Could you check a few things on this model? Use its own coordinates, in mm. A direction names the side the tool comes from. Give positions to 0.01 mm unless a question says otherwise; leave off trailing zeros. Loops run counter-clockwise (first coordinate to the right, second up) from the corner with the lowest first, then second, coordinate; pieces in that order, holes last. Notation, with made-up numbers: M -3.75,-3.5 L 33.25,-3.5 A24 ccw 33.25,16.5 Z; hole C 46,1 d5. An arc over 180 degrees is marked long. Answer in a Markdown table with one row per item. Add a question column.
1. Thinking about a two-plate mould opening in Z: for faces 3 (the flat face through (3, 148, -15)), 4 (the cylindrical face through (16.226, 117.044, -28.521)), 5 (the flat face through (15, 148, 0)), which applies, released by +Z, released by -Z, zero draft, split by the parting line, or undercut?
2. I'm going to push flat-ended pins straight in: pin 1 Ø10 at (y, z) = (254, -4) entering from -X; pin 2 Ø3 at (y, z) = (60, -15) entering from -X. Where does each tip first touch, or does it pass through?
3. If we section it at B-B on x = 23.75: List the corners of the cut face in (y, z) for me, then the cut area to 3 significant figures.
4. If we section it at A-A on y = 140: List the corners of the cut face in (x, z) for me, then the cut area to 3 significant figures.
5. I need wall thicknesses on line 1 along Y through (x, z) = (28.55, -15); line 2 along X through (y, z) = (227.5, -15.25); line 3 along Z through (x, y) = (15.5, 177). Which ranges of each line are inside material? Lowest first, please. Write a range as from..to.
6. Which directions (+Z, -Z, +X, -X, +Y, -Y) give clear straight access to the entire face, cutting with the end or side of a thin tool? Please do faces 1 (the flat face through (15, 148, -3)), 2 (the cylindrical face through (16.226, 117.044, -1.521)).
7. If we section it at D-D on y = 256: List the corners of the cut face in (x, z) for me, then the cut area to 3 significant figures.
8. If we section it at C-C on z = -22.75: List the corners of the cut face in (x, y) for me, then the cut area to 3 significant figures.
Autodesk Inventor part; units mm, degrees
ref_plane "YZ Plane" through (0, 0, 0) normal (1, 0, 0) x (0, 1, 0)
ref_plane "XZ Plane" through (0, 0, 0) normal (0, 1, 0) x (-1, 0, 0)
ref_plane "XY Plane" through (0, 0, 0) normal (0, 0, 1) x (1, 0, 0)
sketch "スケッチ1" plane through (0, 0, 0) normal (0, 1, 0) x (-1, 0, 0)
  line L0 (0, 0) -> (-30, 0)
  line L1 (-30, 0) -> (-30, -30)
  line L2 (-30, -30) -> (0, -30)
  line L3 (0, -30) -> (0, 0)
  line L4 (-3, -3) -> (-27, -3)
  line L5 (-27, -3) -> (-27, -27)
  line L6 (-27, -27) -> (-3, -27)
  line L7 (-3, -27) -> (-3, -3)
  dimension "d0" = 30
  dimension "d1" = 30
  dimension "d2" = 24
  dimension "d3" = 24
  dimension "d4" = 3
  dimension "d5" = 3
extrude "押し出し1" add sketch "スケッチ1" along normal blind 300
sketch "スケッチ2" plane through (0, 0, 0) normal (0, 0, 1) x (1, 0, 0)
  point P0 (0, 0)
  point P1 (13.8561, 31.5859)
sketch "スケッチ3" plane through (30, 0, 0) normal (1, 0, 0) x (0, 0, -1)
  line L0 (30, 0) -> (30, 300)
  line L1 (0, 0) -> (30, 0)
  point P0 (15, 60)
  point P1 (15, 30)
  point P2 (15, 0)
  dimension "d11" = 30
  dimension "d12" = 30
hole "穴1" at (30, 30, -15) at (30, 60, -15) direction (-1, 0, 0) diameter 3.2 end through all
sketch "スケッチ4" plane through (0, 0, 0) normal (0, 0, 1) x (1, 0, 0)
  line L0 (30, 0) -> (0, 0) construction
  line L1 (15, 0) -> (15, 300) construction
  line L2 (30, 300) -> (0, 300) construction
  point P0 (15, 120)
  point P1 (15, 140)
  dimension "d20" = 120
  dimension "d21" = 20
hole "穴2" at (15, 120, 0) at (15, 140, 0) direction (0, 0, -1) diameter 6.4 end through all
properties part number "base" material "アルミニウム 6061"
Results:
| question | item | result |
|---|---|---|
| 1 | face 3 | undercut |
| 1 | face 4 | zero draft |
| 1 | face 5 | released by +Z |
| 2 | pin 1 | x = 0 |
| 2 | pin 2 | through |
| 3 | outline | M 0,-30 L 300,-30 L 300,-27 L 0,-27 Z; M 0,-3 L 300,-3 L 300,0 L 0,0 Z |
| 3 | area | 1,800 mm2 |
| 4 | outline | M 0,-30 L 11.8,-30 L 11.8,-27 L 3,-27 L 3,-3 L 11.8,-3 L 11.8,0 L 0,0 Z; M 18.2,-30 L 30,-30 L 30,0 L 18.2,0 L 18.2,-3 L 27,-3 L 27,-27 L 18.2,-27 Z |
| 4 | area | 286 mm2 |
| 5 | line 1 | 0..28.4, 31.6..58.4, 61.6..300 |
| 5 | line 2 | 0..3, 27..30 |
| 5 | line 3 | -30..-27, -3..0 |
| 6 | face 1 | +Y, -Y |
| 6 | face 2 | +Z, -Z |
| 7 | outline | M 0,-30 L 30,-30 L 30,0 L 0,0 Z; hole M 3,-27 L 27,-27 L 27,-3 L 3,-3 Z |
| 7 | area | 324 mm2 |
| 8 | outline | M 0,0 L 3,0 L 3,300 L 0,300 Z; M 27,0 L 30,0 L 30,300 L 27,300 Z |
| 8 | area | 1,800 mm2 |
